Geometry check sheet. Reference: the model listing, model coordinates, mm. A direction names the side the tool comes from. Give positions to 0.01 mm unless a question says otherwise; leave off trailing zeros. Loops run counter-clockwise (first coordinate to the right, second up) from the corner with the lowest first, then second, coordinate; pieces in that order, holes last. Notation, with made-up numbers: (21, 81.5) -> (33, 81.5) arc R22 cw to (33, 96.5) -> close; hole circle Ø9 at (63, 18.5). An arc over 180 degrees is marked (long way). One line per item, written item: value. Start each with the question number.
(1) Sectioned sample at B-B, the plane x = 0. Record the cut outline in (y, z), then the cut area to 3 significant figures.
(2) Tool access check on faces 4 (the face through (-24.4, -2.03, 14.43)), 5 (the face through (-2.17, -8.93, 9.76)). Record the directions out of +Z, -Z, +X, -X, +Y, -Y that give a thin tool (end or side, any length) a straight path to the whole face; none if there is none.
(3) Draft check along X on faces 1 (the face through (-7.493, -12.986, -0.33)), 2 (the face through (25, -2, 0)), 3 (the face through (7, -14, -4)). Enter one of: pulls with the +X half, pulls with the -X half, needs draft (parallel to the pull), parting line crosses it, or undercut.
(4) Sectioned sample at D-D, the plane z = 9.5. Record the cut outline in (x, y).
(5) Scan lines: line 1 along Z through (x, y) = (0, -13.45); line 2 along Y through (x, z) = (10, 4.5); line 3 along Y through (x, z) = (0, -1). Record each from-to range of solid material in increasing order. Write a range as from..to.
(6) Gauge pin test, flat ends, axial feed: pin 1 Ø1 at (y, z) = (-10.5, 5) entering from +X; pin 2 Ø3 at (y, z) = (-10.5, -8.5) entering from -X; pin 3 Ø1 at (x, z) = (12.5, -9) entering from -Y. Record the tip position at first contact, or that the pin passes through.
(7) Sectioned sample at C-C, the plane y = -7.75. Record the cut outline in (x, z), then the cut area to 3 significant figures.
(8) Sectioned sample at A-A, the plane z = -6. Record the cut outline in (x, y), then the cut area to 3 significant figures.
Solid Edge part; units mm, degrees
sketch "Sketch1" plane through (0, 0, 0) normal (0, -1, 0) x (1, 0, 0)
  line L0 (25, -15) -> (25, 15)
  line L1 (25, 15) -> (-25, 15)
  line L2 (-25, 15) -> (-25, -15)
  line L3 (-25, -15) -> (25, -15)
extrude "Protrusion1" add sketch "Sketch1" along normal blind 4
sketch "Sketch2" plane through (0, -4, 0) normal (0, -1, 0) x (1, 0, 0)
  circle A0 centre (0, 0) radius 7.5
extrude "ExtrudedProtrusion_2" add sketch "Sketch2" along normal blind 8
sketch "Sketch3" plane through (0, -4, 0) normal (0, -1, 0) x (1, 0, 0)
  circle A0 centre (0, 0) radius 10
  circle A1 centre (0, 0) radius 7.5
extrude "ExtrudedProtrusion_3" add sketch "Sketch3" along normal blind 10
fillet "Round_1" radius 2 4 edges at (25, -2, 15) (25, -2, -15) (-25, -2, -15) (-25, -2, 15)
Calculated:
1. outline: (-14, -10) -> (-4, -10) -> (-4, -15) -> (0, -15) -> (0, 15) -> (-4, 15) -> (-4, 10) -> (-14, 10) -> (-14, 7.5) -> (-12, 7.5) -> (-12, -7.5) -> (-14, -7.5) -> close
1. area: 290 mm2
2. face 4: +Z, -X, +Y, -Y
2. face 5: -Y
3. face 1: undercut
3. face 2: pulls with the +X half
3. face 3: needs draft
4. outline: (-25, -4) -> (-3.12, -4) -> (-3.12, -14) -> (3.12, -14) -> (3.12, -4) -> (25, -4) -> (25, 0) -> (-25, 0) -> close
5. line 1: z = -10..-7.5, 7.5..10
5. line 2: y = -4..0
5. line 3: y = -12..0
6. pin 1: stops at x = 8.93
6. pin 2: stops at x = -7.14
6. pin 3: stops at y = -4
7. outline: circle Ø20 at (0, 0)
7. area: 314 mm2
8. outline: (-25, -4) -> (-8, -4) -> (-8, -14) -> (-4.5, -14) -> (-4.5, -12) -> (4.5, -12) -> (4.5, -14) -> (8, -14) -> (8, -4) -> (25, -4) -> (25, 0) -> (-25, 0) -> close
8. area: 342 mm2
